The listing builds one solid part. Answer for the finished solid, in the listing's coordinates (mm). Face numbers are marked on the shaded views. Round coordinates to 2 decimals unless told otherwise and drop trailing zeros. Order: outer loops, then holes, each group sorted by start corner. A loop starts at its lowest first (then second) coordinate and runs counter-clockwise, first axis right, second up. Notation, with made-up numbers: M 70.5,1 L 89.5,1 A11 cw 89.5,14 Z; hole C 89.5,26 d8. An arc over 180 degrees is marked long. Write item = value, one per line. Start each with the question number.
(1) A cutting plane is placed at B-B, the plane y = 14.75. Determine the outline of the cut face in (x, z).
(2) For a pull along X with two mould halves and no side action, classify the marked faces 1, 2, 3 and 4 as released by +X, released by -X, zero draft, split by the parting line, or undercut.
(3) Straight lines are drawn through the part: probe 1 along X at (y, z) = (14.5, 2); probe 2 along X at (y, z) = (15.75, 3.5); probe 3 along Z at (x, y) = (-35.5, 18.25). For each, find the intervals that lie inside material, in ascending order. Write a range as from..to.
(4) Each of these flat-tipped pins is pushed along its axis until it touches: pin 1 (2 mm diameter, centred on x = -43.5, y = 18.5, fed in from -Z); pin 2 (3 mm diameter, centred on x = -36.93, z = 7.5, fed in from +Y). Where does it stop, or does it pass through?
(5) A cutting plane is placed at A-A, the plane z = 7.5. Determine the outline of the cut face in (x, y), and give its area (3 significant figures).
(6) A cutting plane is placed at D-D, the plane z = 3. Determine the outline of the cut face in (x, y).
(7) A cutting plane is placed at C-C, the plane y = 17. Determine the outline of the cut face in (x, z), and give its area (3 significant figures).
from build123d import *

# Parameters (mm, degrees)
F1_DEPTH = 15
F2_R     = 1.6
F3_DEPTH = 7


with BuildPart() as f1:
    # F0 (on Top) → F1 (new body)
    with BuildSketch(Plane.XY):
        with BuildLine():
            Line((-21.92891, 20.478352), (-51.92891, 20.478352))
            Line((-51.92891, 20.478352), (-51.92891, 14.23985))
            Line((-51.92891, 14.23985), (-47.449946, 14.23985))
            ThreePointArc((-47.449946, 14.23985), (-44.42891, 16.252193), (-41.407874, 14.23985))
            Line((-41.407874, 14.23985), (-32.449946, 14.23985))
            ThreePointArc((-32.449946, 14.23985), (-29.42891, 16.252193), (-26.407874, 14.23985))
            Line((-26.407874, 14.23985), (-21.92891, 14.23985))
            Line((-21.92891, 14.23985), (-21.92891, 20.478352))
        make_face()
    extrude(amount=F1_DEPTH)

    # F2 (on face) → F3 (cut)
    with BuildSketch(Plane(origin=(0, 20.478352, 0), x_dir=(-1, 0, 0), z_dir=(0, 1, 0))):
        with Locations((36.92891, 7.5)):
            Circle(F2_R)
    extrude(amount=-F3_DEPTH, mode=Mode.SUBTRACT)


solid = f1.part
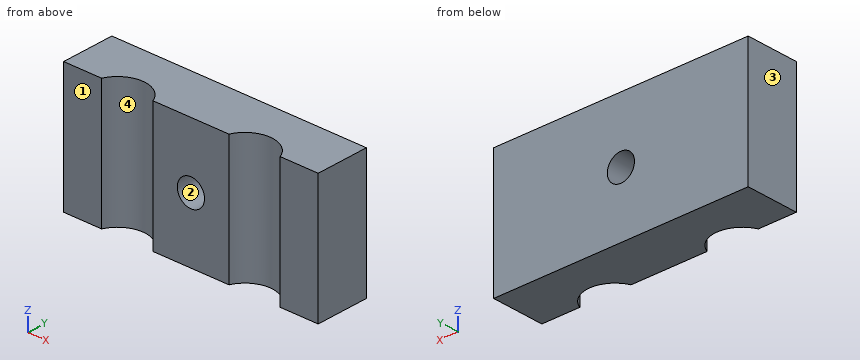
Reported:
q1.outline = M -51.93,0 L -47.18,0 L -47.18,15 L -51.93,15 Z; M -41.68,0 L -32.18,0 L -32.18,15 L -41.68,15 Z; M -26.68,0 L -21.93,0 L -21.93,15 L -26.68,15 Z; hole C -36.93,7.5 d3.2
q2.face_1 = zero draft
q2.face_2 = undercut
q2.face_3 = released by -X
q2.face_4 = undercut
q3.probe_1 = -51.93..-47.33, -41.53..-32.33, -26.53..-21.93
q3.probe_2 = -51.93..-46.17, -42.69..-31.17, -27.69..-21.93
q3.probe_3 = 0..6.78, 8.22..15
q4.pin_1 = 0
q4.pin_2 = through
q5.outline = M -51.93,14.24 L -47.45,14.24 A3.27 cw -41.41,14.24 L -38.53,14.24 L -38.53,20.48 L -51.93,20.48 Z; M -35.33,14.24 L -32.45,14.24 A3.27 cw -26.41,14.24 L -21.93,14.24 L -21.93,20.48 L -35.33,20.48 Z
q5.area = 150 mm²
q6.outline = M -51.93,14.24 L -47.45,14.24 A3.27 cw -41.41,14.24 L -32.45,14.24 A3.27 cw -26.41,14.24 L -21.93,14.24 L -21.93,20.48 L -51.93,20.48 Z
q7.outline = M -51.93,0 L -21.93,0 L -21.93,15 L -51.93,15 Z; hole C -36.93,7.5 d3.2
q7.area = 442 mm²
